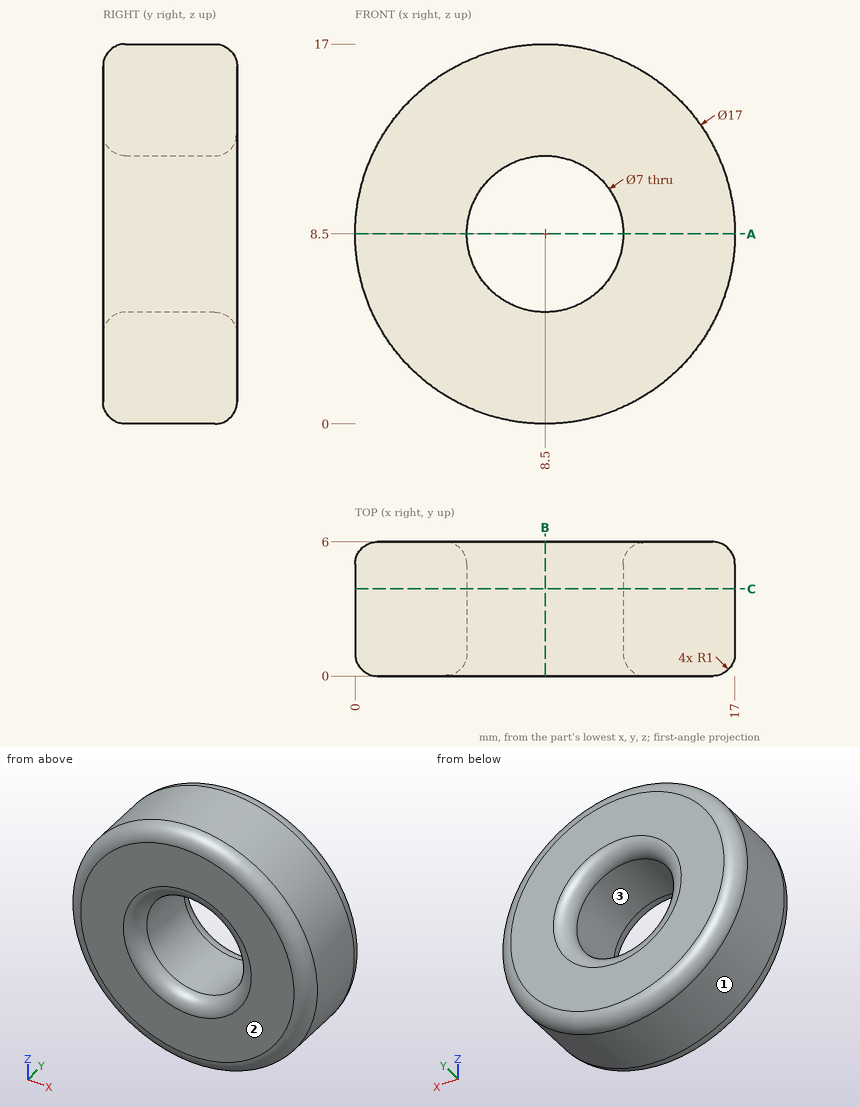
Drawing for the job (mm, zero at the part's lowest x, y, z). Round coordinates to 2 decimals unless told otherwise and drop trailing zeros. Loops run counter-clockwise (first coordinate to the right, second up) from the corner with the lowest first, then second, coordinate; pieces in that order, holes last. Notation, with made-up numbers: (18, 42.25) - (73, 42.25) arc R8 cw to (73, 50.25) - close; hole circle Ø7 at (5, -28). An arc over 180 degrees is marked (long way). Return JSON: item names as keys, results as strings. Group by question number.
Q1. Two-plate mould, pull along Z, no slides. Class the marked faces 1, 2 and 3: +Z half, -Z half, draft (parallel to the pull), parting line (faces both ways), or undercut.
Q2. Band-saw the part on B-B on x = 8.5. Give the cut face in (y, z).
Q3. Band-saw the part on C-C on y = 3.9. Give the cut face in (x, z).
Q4. Flat gauge pins, fed straight in: pin 1 Ø2 at (x, y) = (8, 4.5) entering from +Z; pin 2 Ø2 at (y, z) = (2.5, 11.5) entering from +X; pin 3 Ø1 at (x, y) = (5, 3) entering from +Z; pin 4 Ø3 at (y, z) = (2, 5.5) entering from +X. Where does each tip first touch, or does it go through?
Q5. Band-saw the part on A-A on z = 8.5. Give the cut face in (x, y).
Q6. Drill centre lines: line 1 along X through (y, z) = (4.05, 8.5); line 2 along Z through (x, y) = (10.75, 3.3); line 3 along Z through (x, y) = (8.75, 0.3). Where is each one in solid material? Low to high. Write a range as [from, to].
Solutions:
{
 "1": {"face 1": "parting line", "face 2": "draft", "face 3": "undercut"},
 "2": {"outline": "(0, 1) arc R1 ccw to (1, 0) - (5, 0) arc R1 ccw to (6, 1) - (6, 4) arc R1 ccw to (5, 5) - (1, 5) arc R1 ccw to (0, 4) - close; (0, 13) arc R1 ccw to (1, 12) - (5, 12) arc R1 ccw to (6, 13) - (6, 16) arc R1 ccw to (5, 17) - (1, 17) arc R1 ccw to (0, 16) - close"},
 "3": {"outline": "circle Ø17 at (8.5, 8.5); hole circle Ø7 at (8.5, 8.5)"},
 "4": {"pin 1": "stops at z = 17", "pin 2": "stops at x = 16.76", "pin 3": "stops at z = 16.45", "pin 4": "stops at x = 16.87"},
 "5": {"outline": "(0, 1) arc R1 ccw to (1, 0) - (4, 0) arc R1 ccw to (5, 1) - (5, 5) arc R1 ccw to (4, 6) - (1, 6) arc R1 ccw to (0, 5) - close; (12, 1) arc R1 ccw to (13, 0) - (16, 0) arc R1 ccw to (17, 1) - (17, 5) arc R1 ccw to (16, 6) - (13, 6) arc R1 ccw to (12, 5) - close"},
 "6": {"line 1": "x = [0, 5], [12, 17]", "line 2": "z = [0.3, 5.82], [11.18, 16.7]", "line 3": "z = [0.29, 4.72], [12.28, 16.71]"}
}
